```python
from build123d import *

# Parameters (mm, degrees)
SKETCH1_R              = 4.699
BOSS_EXTRUDE1_DEPTH    = 44.45
CUT_SWEEP1_PITCH       = 1.27
CUT_SWEEP1_HEIGHT      = 114.3
CUT_SWEEP1_RADIUS      = 4.699
CUT_SWEEP1_START_ANGLE = -90
SKETCH4_W              = 4.69845619
SKETCH4_H              = 16.911386709
SKETCH5_W              = 0.723886717
SKETCH5_H              = 17.397939395
SKETCH6_R              = 2.794
CUT_EXTRUDE1_DEPTH     = 6.35
CHAMFER1_SIZE          = 0.508
CHAMFER2_SIZE          = 0.79375
CHAMFER2_SIZE2         = 0.567023999
CHAMFER2_EDGE_2_SIZE   = 0.79375
CHAMFER2_EDGE_2_SIZE2  = 0.567023999
FILLET1_R              = 0.762
CHAMFER3_SIZE          = 0.3048
FILLET3_R              = 0.508


with BuildPart() as part:
    # Sketch1 → Boss-Extrude1 (new, symmetric)
    with BuildSketch(Plane(origin=(0, 0, 0), x_dir=(1, 0, 0), z_dir=(0, 1, 0))):
        with Locations(Location((0, 0, 0), (0, 0, 270))):
            Circle(SKETCH1_R)
    extrude(amount=BOSS_EXTRUDE1_DEPTH, both=True)

    # Cut-Sweep1: sweep along a helix
    with BuildLine() as cut_sweep1_path:
        add(Helix(CUT_SWEEP1_PITCH, CUT_SWEEP1_HEIGHT, CUT_SWEEP1_RADIUS, center=(0, 44.45, 0), direction=(0, -1, 0), mode=Mode.PRIVATE).rotate(Axis((0, 44.45, 0), (0, -1, 0)), CUT_SWEEP1_START_ANGLE))
    # Sketch3 → Cut-Sweep1 (sweep, cut)
    with BuildSketch(Plane.XY):
        Polygon((-3.99161, 44.606186444), (-3.99161, 44.288686444), (-4.698612835, 43.880498167), (-4.698612835, 45.014374721), align=None)
    sweep(path=cut_sweep1_path.line, is_frenet=True, mode=Mode.SUBTRACT)

    # Sketch4 → Revolve1 (revolve)
    with BuildSketch(Plane.XY):
        with Locations((-2.349228095, 52.905693355)):
            Rectangle(SKETCH4_W, SKETCH4_H)
    revolve(axis=Axis((0, 44.45, 0), (0, 1, 0)))

    # Sketch5 → Cut-Revolve1 (revolve, cut)
    with BuildSketch(Plane.XY):
        with Locations((-5.02318101, 53.148969698)):
            Rectangle(SKETCH5_W, SKETCH5_H)
    revolve(axis=Axis((0, 62.766926139, 0), (0, -1, 0)), mode=Mode.SUBTRACT)

    # Sketch6 → Cut-Extrude1 (cut, symmetric)
    with BuildSketch(Plane.XY):
        with Locations((0, 55.011386709)):
            Circle(SKETCH6_R)
    extrude(amount=CUT_EXTRUDE1_DEPTH, both=True, mode=Mode.SUBTRACT)

    # Chamfer1
    chamfer1_edges = [part.edges().sort_by_distance(p)[0] for p in [
        (4.661237651, 61.361386709, 0),
    ]]
    chamfer(chamfer1_edges, length=CHAMFER1_SIZE)

    # Chamfer2
    chamfer2_edges = [part.edges().sort_by_distance(p)[0] for p in [
        (-2.794, 55.011386706, -3.731045488),
    ]]
    chamfer2_side = [part.faces().sort_by_distance(p)[0] for p in [
        (4.661237651, 52.651693354, 0),
    ]]
    chamfer(chamfer2_edges, length=CHAMFER2_SIZE, length2=CHAMFER2_SIZE2, reference=chamfer2_side[0])

    # Chamfer2 edge 2
    chamfer2_edge_2_edges = [part.edges().sort_by_distance(p)[0] for p in [
        (-2.794, 55.011386706, 3.731045488),
    ]]
    chamfer2_edge_2_side = [part.faces().sort_by_distance(p)[0] for p in [
        (4.661237651, 52.651693354, 0),
    ]]
    chamfer(chamfer2_edge_2_edges, length=CHAMFER2_EDGE_2_SIZE, length2=CHAMFER2_EDGE_2_SIZE2, reference=chamfer2_edge_2_side[0])

    # Sketch7 → Revolve2 (revolve)
    with BuildSketch(Plane.XY):
        with BuildLine():
            Line((-3.98526, -44.45), (0, -44.45))
            Line((0, -44.45), (0, -48.645010112))
            Line((0, -48.645010112), (0, -53.407510112))
            ThreePointArc((0, -53.407510112), (-4.189252508, -50.910306929), (-3.98526, -46.0375))
            Line((-3.98526, -46.0375), (-3.98526, -44.45))
        make_face()
    revolve(axis=Axis((0, -47.823804308, 0), (0, -1, 0)))

    # Sketch8 → Cut-Revolve2 (revolve, cut)
    with BuildSketch(Plane.XY):
        Polygon((3.98526, -46.0375), (3.98526, -44.45), (5.088678737, -43.346581263), (5.088678737, -46.0375), align=None)
    revolve(axis=Axis((0, -56.16584847, 0), (0, 1, 0)), mode=Mode.SUBTRACT)


with BuildPart() as body_2:
    # Sketch9 → Revolve3 (revolve)
    with BuildSketch(Plane.XY):
        with BuildLine():
            Line((4.769366022, -47.907837304), (5.378396166, -47.907837304))
            ThreePointArc((5.378396166, -47.907837304), (5.424274511, -47.985297574), (5.470454774, -48.062578228))
            ThreePointArc((5.470454774, -48.062578228), (6.014262065, -49.72815682), (5.779486953, -51.464462974))
            ThreePointArc((5.779486953, -51.464462974), (6.076106552, -53.860794812), (8.21501488, -54.981268207))
            Line((8.21501488, -54.981268207), (8.855493066, -54.981268207))
            Line((8.855493066, -54.981268207), (8.855493066, -56.22448981))
            Line((8.855493066, -56.22448981), (0, -56.22448981))
            Line((0, -56.22448981), (0, -53.471010112))
            ThreePointArc((0, -53.471010112), (3.663868991, -51.786083179), (4.769366022, -47.907837304))
        make_face()
    revolve(axis=Axis((0, -48.645010112, 0), (0, -1, 0)))

    # Fillet1
    fillet1_edges = [body_2.edges().sort_by_distance(p)[0] for p in [
        (-5.378396166, -47.907837304, 0),
    ]]
    fillet(fillet1_edges, radius=FILLET1_R)

    # Chamfer3
    chamfer3_edges = [body_2.edges().sort_by_distance(p)[0] for p in [
        (-8.855493066, -54.981268207, 0),
    ]]
    chamfer(chamfer3_edges, length=CHAMFER3_SIZE)


with BuildPart() as body_3:
    # Sketch10 → Revolve4 (revolve)
    with BuildSketch(Plane(origin=(0, 0, 0), x_dir=(0, 0, -1), z_dir=(1, 0, 0)), mode=Mode.PRIVATE) as revolve4_sk:
        with BuildLine():
            Line((-25.078931212, 55.011386709), (49.420548196, 55.011386709))
            ThreePointArc((49.420548196, 55.011386709), (47.227520009, 58.284257823), (43.366572257, 57.500586709))
            Line((43.366572257, 57.500586709), (-18.922230923, 57.500586709))
            ThreePointArc((-18.922230923, 57.500586709), (-22.868342697, 58.402277998), (-25.078931212, 55.011386709))
        make_face()
    revolve(revolve4_sk.sketch.rotate(Axis((0, 55.011386709, 6.574e-06), (0, 0, -1)), 90), axis=Axis((0, 55.011386709, 6.574e-06), (0, 0, -1)))

    # Fillet3
    fillet3_edges = [body_3.edges().sort_by_distance(p)[0] for p in [
        (-2.4892, 55.011386709, 18.922230923),
        (-2.4892, 55.011386709, -43.366572257),
    ]]
    fillet(fillet3_edges, radius=FILLET3_R)


solid = body_3.part
```
The model under review builds one solid part; all positions refer to its coordinate system, in mm. Round coordinates to 2 decimals unless told otherwise and drop trailing zeros. Order: outer loops, then holes, each group sorted by start corner. A loop starts at its lowest first (then second) coordinate and runs counter-clockwise, first axis right, second up.
Item 1: To check wall thickness, follow probe 1 along Z at (x, y) = (-0.75, 52.5); probe 2 along Y at (x, z) = (-0.25, 10.5); probe 3 along Z at (x, y) = (-0.75, 57.5). State the ranges of each line that lie inside material, in increasing order.
Working result:
probe 1: z = -48.26 to -43.5, 19.05 to 24.04
probe 2: y = 52.53 to 57.49
probe 3: z = -48.28 to -43.48, 19.02 to 24.06
Item 2: For pin 1 (1 mm diameter, centred on x = -1.5, y = 57.5, fed in from -Z); pin 2 (3 mm diameter, centred on y = 53.5, z = -11, fed in from +X); pin 3 (4 mm diameter, centred on y = 56.5, z = 13.5, fed in from -X), all flat-tipped, find the tip position at first contact; note any pin that passes through.
Working result:
pin 1: stops at z = -48.48
pin 2: stops at x = 2.49
pin 3: stops at x = -2.49
Item 3: Add section A-A, the plane z = -20. State the section outline as (x, y) points.
Working result:
outline: circle Ø4.98 at (0, 55.01)
